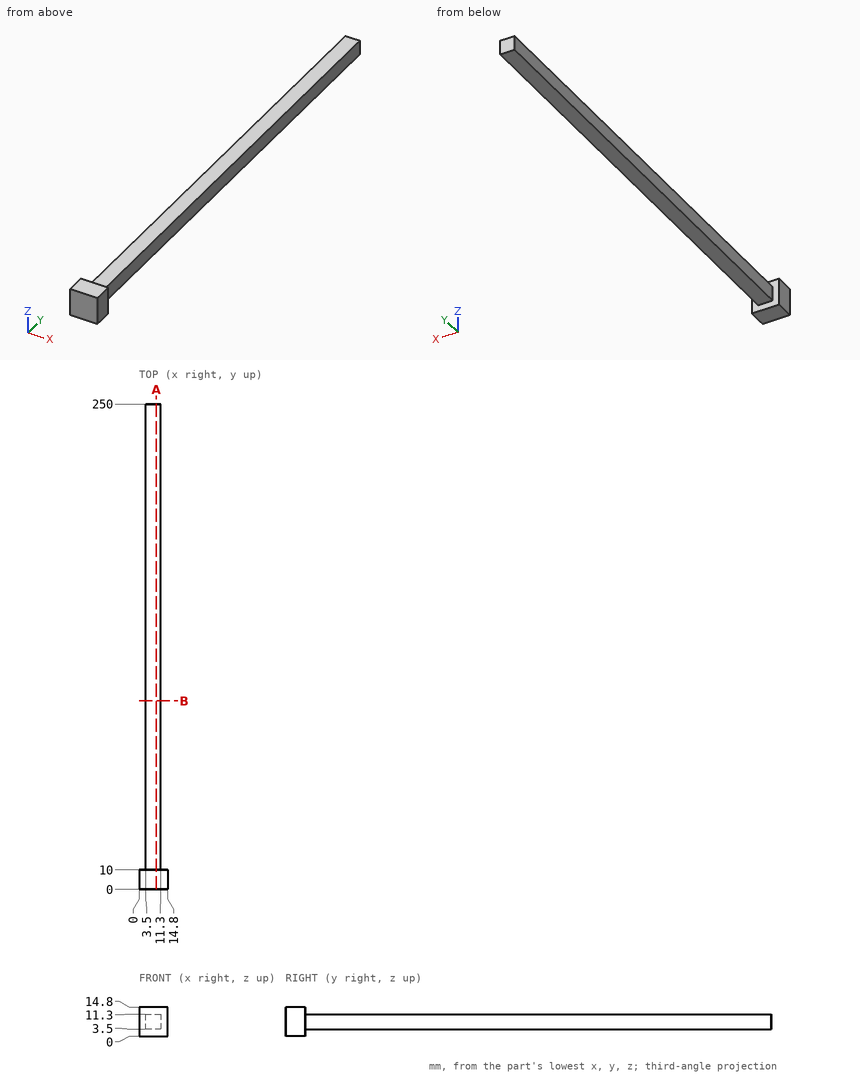
The drawing under review shows one solid part. Ordinate dimensions are in mm from its lowest x, y, z. Give positions to 0.01 mm unless a question says otherwise; leave off trailing zeros. Order: outer loops, then holes, each group sorted by start corner. A loop starts at its lowest first (then second) coordinate and runs counter-clockwise, first axis right, second up. Notation, with made-up numbers: (54, -37) -> (96, -37) arc R18 ccw to (96, -29) -> close; hole circle Ø9 at (22.25, -1.75). An arc over 180 degrees is marked (long way). Write item = value, one per line. Start each with the question number.
(1) We need section B-B on y = 97. Write out the cut boundary in (x, z), plus the area to 3 significant figures.
(2) For pin 1 (4 mm diameter, centred on y = 148, z = 8.5, fed in from -X); pin 2 (1.5 mm diameter, centred on y = 151, z = 6, fed in from +X); pin 3 (1.5 mm diameter, centred on x = 7.5, z = 4.5, fed in from -Y); pin 4 (1.5 mm diameter, centred on x = 6, y = 111.5, fed in from -Z), all flat-tipped, find the tip position at first contact; note any pin that passes through.
(3) We need section A-A on x = 9. Write out the cut boundary in (y, z), plus the area to 3 significant figures.
(4) To check wall thickness, follow line 1 along X through (y, z) = (77.5, 7.5); line 2 along Y through (x, z) = (2.5, 12.5). State the ranges of each line that lie inside material, in increasing order.
Numbers:
q1.outline = (3.5, 3.5) -> (11.3, 3.5) -> (11.3, 11.3) -> (3.5, 11.3) -> close
q1.area = 60.8 mm^2
q2.pin_1 = 3.5
q2.pin_2 = 11.3
q2.pin_3 = 0
q2.pin_4 = 3.5
q3.outline = (0, 0) -> (10, 0) -> (10, 3.5) -> (250, 3.5) -> (250, 11.3) -> (10, 11.3) -> (10, 14.8) -> (0, 14.8) -> close
q3.area = 2,020 mm^2
q4.line_1 = 3.5 to 11.3
q4.line_2 = 0 to 10
